Can you work these out from the model? Positions are in its coordinate system, mm. Face numbers are marked on the shaded views. A direction names the side the tool comes from. Round coordinates to 2 decimals unless told otherwise and drop trailing zeros. Write each loop counter-clockwise with the first axis right and the second up, starting at its lowest first coordinate (ties: lowest second). Pieces come first, ordered by that corner, then holes. Notation, with made-up numbers: (53, 36) - (110, 36) arc R29 cw to (110, 69) - close; hole circle Ø4 at (70, -20). An arc over 180 degrees is marked (long way). One line per item, written item: value. Start each with the question number.
(1) On a 3-axis mill with a long thin cutter (end or side, diameter ignored), from which of +Z, -Z, +X, -X, +Y, -Y can I reach the whole of each face in a straight line? I mean the marked faces 4 and 5. Say none if no direction works.
(2) I want a section at B-B on y = 23.5. List the corners of the cut face in (x, z) for me, plus the area to 3 significant figures.
(3) I want a section at D-D on x = 14. List the corners of the cut face in (y, z) for me, plus the area to 3 significant figures.
(4) If I drill on L1, parallel to X at y = 17, z = -118; L2, parallel to Z at x = -62.5, y = 24.5; L3, parallel to X at y = 31, z = -116, over which ranges is the centre line in solid material (lowest first)? Write a range as from..to.
(5) Thinking about a two-plate mould opening in X: for the marked faces 1, 2 and 3, which applies, +X half, -X half, draft (parallel to the pull), parting line (faces both ways), or undercut?
(6) I want a section at A-A on z = -118. List the corners of the cut face in (x, y) for me, plus the area to 3 significant figures.
(7) I'm going to push flat-ended pins straight in: pin 1 Ø4 at (y, z) = (4.5, -36.5) entering from -X; pin 2 Ø12 at (x, y) = (-71.5, 7) entering from -Z; pin 3 Ø1 at (y, z) = (7.5, -35.5) entering from +X. Where does each tip first touch, or does it pass through?
(8) I want a section at C-C on x = 62.5. List the corners of the cut face in (y, z) for me, plus the area to 3 significant figures.
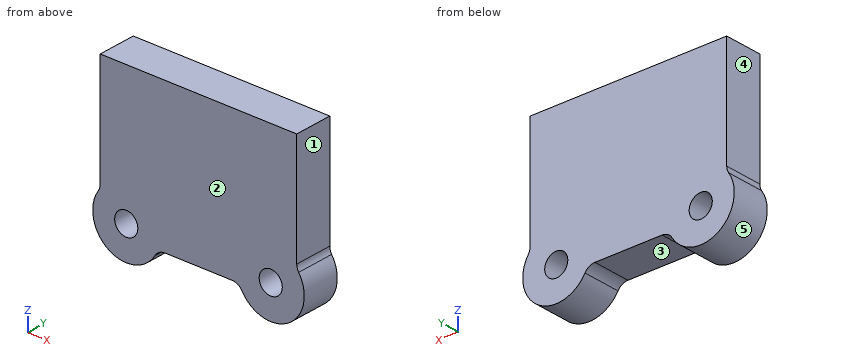
from build123d import *

# Parameters (mm, degrees)
SKETCH1_R           = 10
BOSS_EXTRUDE1_DEPTH = 33
FILLET1_R           = 10


with BuildPart() as part:
    # Sketch1 → Boss-Extrude1 (new body)
    with BuildSketch(Plane(origin=(0, 0, 0), x_dir=(1, 0, 0), z_dir=(0, 1, 0))):
        with BuildLine():
            Line((85, 0), (-85, 0))
            Line((-85, 0), (-85, 99.703825536))
            ThreePointArc((-85, 99.703825536), (-76.843677233, 143.204343345), (-35.278684822, 128))
            Line((-35.278684822, 128), (35.278684822, 128))
            ThreePointArc((35.278684822, 128), (76.843677233, 143.204343345), (85, 99.703825536))
            Line((85, 99.703825536), (85, 0))
        make_face()
        with Locations((-62.5, 118)):
            Circle(SKETCH1_R, mode=Mode.SUBTRACT)
        with Locations((62.5, 118)):
            Circle(SKETCH1_R, mode=Mode.SUBTRACT)
    extrude(amount=BOSS_EXTRUDE1_DEPTH)

    # Fillet1
    fillet1_edges = [part.edges().sort_by_distance(p)[0] for p in [
        (-85, 16.5, -99.703825536),
        (-35.278684822, 16.5, -128),
        (35.278684822, 16.5, -128),
        (85, 16.5, -99.703825536),
    ]]
    fillet(fillet1_edges, radius=FILLET1_R)


solid = part.part
Established:
1. face 4: +Z, -X, +Y, -Y
1. face 5: +Y, -Y
2. outline: (-86.67, -101.97) arc R29 ccw (long way) to (-37.6, -132.87) arc R10 cw to (-29.02, -128) - (29.02, -128) arc R10 cw to (37.6, -132.87) arc R29 ccw (long way) to (86.67, -101.97) arc R10 cw to (85, -96.44) - (85, 0) - (-85, 0) - (-85, -96.44) arc R10 cw to start; hole circle Ø20 at (-62.5, -118); hole circle Ø20 at (62.5, -118)
2. area: 22,900 mm2
3. outline: (0, -128) - (33, -128) - (33, 0) - (0, 0) - close
3. area: 4,220 mm2
4. L1: -91.5..-72.5, -52.5..52.5, 72.5..91.5
4. L2: -147..-128, -108..0
4. L3: -91.43..-72.3, -52.7..52.7, 72.3..91.43
5. face 1: +X half
5. face 2: draft
5. face 3: undercut
6. outline: (-91.5, 0) - (-72.5, 0) - (-72.5, 33) - (-91.5, 33) - close; (-52.5, 0) - (52.5, 0) - (52.5, 33) - (-52.5, 33) - close; (72.5, 0) - (91.5, 0) - (91.5, 33) - (72.5, 33) - close
6. area: 4,720 mm2
7. pin 1: x = -85
7. pin 2: z = -146.84
7. pin 3: x = 85
8. outline: (0, -147) - (33, -147) - (33, -128) - (0, -128) - close; (0, -108) - (33, -108) - (33, 0) - (0, 0) - close
8. area: 4,190 mm2
